Can you work these out from the model? Positions are in its coordinate system, mm. Face numbers are marked on the shaded views. A direction names the side the tool comes from. Round coordinates to 2 decimals unless told otherwise and drop trailing zeros.
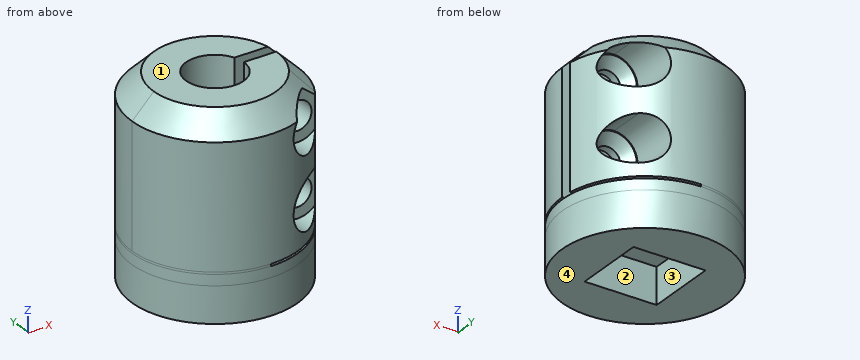
from build123d import *
from build123d.topology import SkipClean

# Parameters (mm, degrees)
SZKIC1_R                                           = 11.5
SZKIC1_R_2                                         = 4
DODANIE_WYCI_GNI_CIE1_DEPTH                        = 20
SZKIC3_W                                           = 11.5
SZKIC3_H                                           = 20
WYTNIJ_WYCI_GNI_CIE1_DEPTH                         = 1.5
WYTNIJ_WYCI_GNI_CIE2_DEPTH                         = 32
POG_BIENIE_STO_KOWE_POD_M3_WKR_T_Z_BEM_D           = 3.6
POG_BIENIE_STO_KOWE_POD_M3_WKR_T_Z_BEM_CSINK_D     = 6.3
POG_BIENIE_STO_KOWE_POD_M3_WKR_T_Z_BEM_CSINK_ANGLE = 90
SZKIC7_R                                           = 3.5
WYTNIJ_WYCI_GNI_CIE3_DEPTH                         = 32
SZKIC8_R                                           = 2
WYTNIJ_WYCI_GNI_CIE4_DEPTH                         = 7
DODANIE_WYCI_GNI_CIE2_START                        = 0.3
DODANIE_WYCI_GNI_CIE2_DEPTH                        = 0.3
DODANIE_WYCI_GNI_CIE3_START                        = 1.5
SZKIC10_R                                          = 11.5
DODANIE_WYCI_GNI_CIE3_DEPTH                        = 1.5
DODANIE_WYCI_GNI_CIE4_START                        = 5
SZKIC11_R                                          = 11.5
SZKIC11_W                                          = 10
SZKIC11_H                                          = 10
DODANIE_WYCI_GNI_CIE4_DEPTH                        = 5
SFAZOWANIE1_SIZE                                   = 3


with BuildPart() as part:
    # Szkic1 → Dodanie-wyciągnięcie1 (new body)
    with BuildSketch(Plane.XY):
        with Locations(Location((0, 0, 0), (0, 0, 180))):
            Circle(SZKIC1_R)
        with Locations(Location((0, 0, 0), (0, 0, 180))):
            Circle(SZKIC1_R_2, mode=Mode.SUBTRACT)
    extrude(amount=DODANIE_WYCI_GNI_CIE1_DEPTH)

    # Szkic3 → Wytnij-wyciągnięcie1 (cut)
    with BuildSketch(Plane(origin=(0, 0, 0), x_dir=(1, 0, 0), z_dir=(0, 1, 0))):
        with Locations((5.75, -10)):
            Rectangle(SZKIC3_W, SZKIC3_H)
    extrude(amount=WYTNIJ_WYCI_GNI_CIE1_DEPTH, mode=Mode.SUBTRACT)

    # Szkic4 → Wytnij-wyciągnięcie2 (cut)
    with BuildSketch(Plane(origin=(0, 4, 0), x_dir=(1, 0, 0), z_dir=(0, 1, 0))):
        with BuildLine():
            ThreePointArc((7, -11.75), (3.75, -15), (7, -18.25))
            Line((7, -18.25), (7, -11.75))
        make_face()
        with BuildLine():
            Line((7, -11.75), (7, -18.25))
            ThreePointArc((7, -18.25), (9.298097039, -17.298097039), (10.25, -15))
            ThreePointArc((10.25, -15), (9.298097039, -12.701902961), (7, -11.75))
        make_face()
        with BuildLine():
            ThreePointArc((7, -1.75), (3.75, -5), (7, -8.25))
            Line((7, -8.25), (7, -1.75))
        make_face()
        with BuildLine():
            Line((7, -1.75), (7, -8.25))
            ThreePointArc((7, -8.25), (9.298097039, -7.298097039), (10.25, -5))
            ThreePointArc((10.25, -5), (9.298097039, -2.701902961), (7, -1.75))
        make_face()
    extrude(amount=WYTNIJ_WYCI_GNI_CIE2_DEPTH, mode=Mode.SUBTRACT)

    # Pogłębienie stożkowe pod M3 Wkręt z łbem płaskim1 (through all)
    with Locations(Plane(origin=(7, 4, 15), x_dir=(0, 0, 1), z_dir=(0, 1, 0))):
        with Locations((0, 0), (-10, 0)):
            CounterSinkHole(POG_BIENIE_STO_KOWE_POD_M3_WKR_T_Z_BEM_D / 2, POG_BIENIE_STO_KOWE_POD_M3_WKR_T_Z_BEM_CSINK_D / 2, counter_sink_angle=POG_BIENIE_STO_KOWE_POD_M3_WKR_T_Z_BEM_CSINK_ANGLE)

    # Szkic7 → Wytnij-wyciągnięcie3 (cut)
    with BuildSketch(Plane(origin=(0, -6.5, 0), x_dir=(-1, 0, 0), z_dir=(0, -1, 0))):
        with Locations((-7, -5)):
            Circle(SZKIC7_R)
        with Locations((-7, -15)):
            Circle(SZKIC7_R)
    extrude(amount=WYTNIJ_WYCI_GNI_CIE3_DEPTH, mode=Mode.SUBTRACT)

    # Szkic8 → Wytnij-wyciągnięcie4 (cut)
    with BuildSketch(Plane.XZ.offset(6.5)):
        with Locations((7, 15)):
            Circle(SZKIC8_R)
        with Locations(Location((7, 5, 0), (0, 0, 90))):
            Circle(SZKIC8_R)
    extrude(amount=-WYTNIJ_WYCI_GNI_CIE4_DEPTH, mode=Mode.SUBTRACT)

    # Szkic9 → Dodanie-wyciągnięcie2 (add)
    with SkipClean():  # the faces are left unmerged after this step: merging them gives an invalid solid
        with BuildSketch(Plane(origin=(0, 0, 0), x_dir=(-1, 0, 0), z_dir=(0, 0, -1)).offset(DODANIE_WYCI_GNI_CIE2_START)):
            with BuildLine():
                Line((0, 11.5), (0, 4))
                ThreePointArc((0, 4), (4, 0), (0, -4))
                Line((0, -4), (0, -11.5))
                ThreePointArc((0, -11.5), (11.5, 0), (0, 11.5))
            make_face()
        extrude(amount=-DODANIE_WYCI_GNI_CIE2_DEPTH)

    # Szkic10 → Dodanie-wyciągnięcie3 (add)
    with SkipClean():  # the faces are left unmerged after this step: merging them gives an invalid solid
        with BuildSketch(Plane(origin=(0, 0, -0.3), x_dir=(-1, 0, 0), z_dir=(0, 0, -1)).offset(DODANIE_WYCI_GNI_CIE3_START)):
            Circle(SZKIC10_R)
        extrude(amount=-DODANIE_WYCI_GNI_CIE3_DEPTH)

    # Szkic11 → Dodanie-wyciągnięcie4 (add)
    with SkipClean():  # the faces are left unmerged after this step: merging them gives an invalid solid
        with BuildSketch(Plane(origin=(0, 0, -1.8), x_dir=(-1, 0, 0), z_dir=(0, 0, -1)).offset(DODANIE_WYCI_GNI_CIE4_START)):
            Circle(SZKIC11_R)
            Rectangle(SZKIC11_W, SZKIC11_H, mode=Mode.SUBTRACT)
        extrude(amount=-DODANIE_WYCI_GNI_CIE4_DEPTH)

    # Sfazowanie1
    # the kernel refuses this chamfer: 3 mm, written as the material it takes off along each edge
    with BuildSketch(Plane(origin=(0, 0, 20), x_dir=(-1, 0, 0), z_dir=(0, 1, 0))) as sfazowanie1_piece_1:
        Polygon((11.5, -SFAZOWANIE1_SIZE), (11.5 - SFAZOWANIE1_SIZE, 0), (11.5, 0), align=None)
    revolve(axis=Axis((0, 0, 20), (0, 0, 1)), revolution_arc=218.500054596, mode=Mode.SUBTRACT)
    with BuildSketch(Plane(origin=(0, 0, 20), x_dir=(0.8571646812696857, -0.5150424343525863, 0), z_dir=(-0.5150424343525863, -0.8571646812696857, 0))) as sfazowanie1_piece_2:
        Polygon((11.5, -SFAZOWANIE1_SIZE), (11.5 - SFAZOWANIE1_SIZE, 0), (11.5, 0), align=None)
    revolve(axis=Axis((0, 0, 20), (0, 0, 1)), revolution_arc=211.000291399, mode=Mode.SUBTRACT)


solid = part.part
(1) For the marked faces 1 and 2, which set-ups out of +Z, -Z, +X, -X, +Y, -Y let a thin tool reach every point of the face, with its end or its side?
Worked answers:
face 1: +Z, +X, -X, +Y, -Y
face 2: -Z
(2) If we mould it in two halves opening along X, with no side actions, what happens to the marked faces 3 and 4? For each: released by +X, released by -X, zero draft, split by the parting line, or undercut.
Worked answers:
face 3: undercut
face 4: zero draft
(3) Will these pins go through, and if not, where does the flat tip stop? P1, Ø3, axis at x = 6.5, z = 17, coming from the +Y side; P2, Ø2.5, axis at y = -2, z = -5.5, coming from the -X side; P3, Ø3, axis at x = -0.5, y = 2.5, coming from the -Z side.
Worked answers:
P1: stops at y = 9.51
P2: stops at x = -11.48
P3: stops at z = -1.8
(4) If we section it at A-A, the plane y = 3: State how many separate pieces and enclosed holes the cut face has, then the cut area to 3 significant figures.
Worked answers:
separate pieces: 2
enclosed holes: 2
area: 397 mm2
(5) If I drill on line 1 (Z direction, x = 7, y = 2.4); line 2 (X direction, y = 1.85, z = 5); line 3 (Z direction, x = 7, y = -7.8), over which ranges is the centre line in solid material (lowest first)?
Worked answers:
line 1: z = -6.8 to -0.3, 0 to 3.2, 6.8 to 13.2, 16.8 to 20
line 2: x = -11.35 to -3.55, 3.55 to 5.2, 8.8 to 11.35
line 3: z = -6.8 to -0.3, 0 to 1.5, 8.5 to 11.5
